from build123d import *

# Parameters (mm, degrees)
BOSS_EXTRUDE1_DEPTH = 60.96
CUT_EXTRUDE1_REACH  = 147.095
SKETCH3_W           = 40.961637843
SKETCH3_H           = 33.750081885


with BuildPart() as part:
    # Sketch1 → Boss-Extrude1 (new body)
    with BuildSketch(Plane(origin=(0, 0, 0), x_dir=(1, 0, 0), z_dir=(0, 1, 0))):
        with BuildLine():
            ThreePointArc((92.976117224, 4.860881604), (-74.724124634, 55.538200742), (22.152321734, -90.429315965))
            ThreePointArc((22.152321734, -90.429315965), (24.083056487, -17.899569011), (92.976117224, 4.860881604))
        make_face()
    extrude(amount=BOSS_EXTRUDE1_DEPTH)

    # Sketch3 → Cut-Extrude1 (cut, up to next)
    with BuildSketch(Plane(origin=(0, 60.96, 0), x_dir=(1, 0, 0), z_dir=(0, 1, 0)), mode=Mode.PRIVATE) as cut_extrude1_sk1:
        with Locations((-100.15988625, -50.336660589)):
            Rectangle(SKETCH3_W, SKETCH3_H)
    cut_extrude1_tool1 = extrude(cut_extrude1_sk1.sketch, amount=-CUT_EXTRUDE1_REACH, mode=Mode.PRIVATE) & part.part
    add(cut_extrude1_tool1.solids().sort_by_distance((-100.159886, 60.96, 50.336661))[0], mode=Mode.SUBTRACT)


solid = part.part
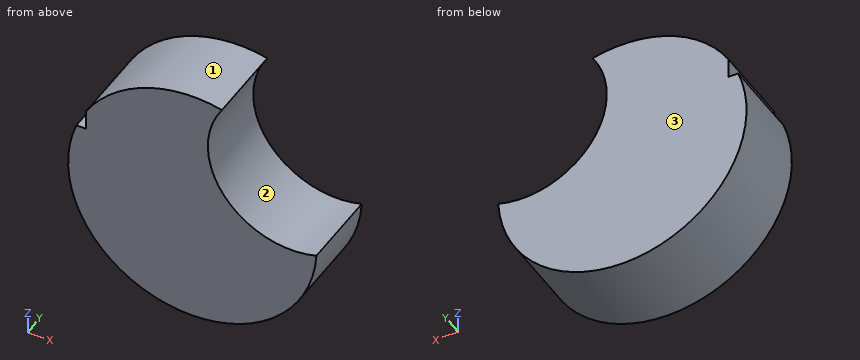
Work out the finished part from the listing and answer in its coordinate system (mm). Face numbers are marked on the shaded views. Give positions to 0.01 mm unless a question says otherwise; leave off trailing zeros. Order: outer loops, then holes, each group sorted by start corner. A loop starts at its lowest first (then second) coordinate and runs counter-clockwise, first axis right, second up. Notation, with made-up numbers: (74.25, -34) -> (86.25, -34) arc R20 ccw to (86.25, -15) -> close; hole circle Ø5 at (82.5, 67). An arc over 180 degrees is marked (long way). Answer as a JSON object with one key per item and string values. Group by question number.
1. The mould has two halves that part along Z. Classify the marked faces 1, 2 and 3: released by +Z, released by -Z, zero draft, split by the parting line, or undercut.
2. Section B-B on x = -62 is taken. Determine the outline of the cut face in (y, z).
3. Section A-A on z = -64 is taken. Determine the outline of the cut face in (x, y).
4. Flat-ended cylindrical pins translate along their axes: pin 1 Ø5 at (y, z) = (12, -58.5) entering from -X; pin 2 Ø8 at (x, y) = (-84, 40.5) entering from +Z; pin 3 Ø1 at (y, z) = (41.5, 16.5) entering from -X. Find the tip coordinate at first contact, or state that the pin passes through.
5. Section C-C on y = 50 is taken. Determine the outline of the cut face in (x, z), plus the area to 3 significant figures.
6. Consider line 1 along Z through (x, y) = (-1, 44.5); line 2 along X through (y, z) = (23.5, 55.5); line 3 along X through (y, z) = (10, -78). Determine where each line is inside the solid, lowest interval first. Write a range as [from, to].
Result sheet:
{
 "1": {"face 1": "released by +Z", "face 2": "undercut", "face 3": "zero draft"},
 "2": {"outline": "(0, -69.46) -> (60.96, -69.46) -> (60.96, 69.46) -> (0, 69.46) -> close"},
 "3": {"outline": "(-67.62, 0) -> (67.62, 0) -> (67.62, 60.96) -> (-67.62, 60.96) -> close"},
 "4": {"pin 1": "stops at x = -74.38", "pin 2": "stops at z = 33.46", "pin 3": "stops at x = -91.72"},
 "5": {"outline": "(-86.88, 33.46) arc R93.1 ccw (long way) to (92.98, -4.86) arc R63.1 cw to (22.15, 90.43) arc R93.1 ccw to (-79.68, 48.16) -> (-79.68, 33.46) -> close", "area": "21,800 mm^2"},
 "6": {"line 1": "z = [-93.1, 93.1]", "line 2": "x = [-74.75, 11.63]", "line 3": "x = [-50.83, 50.83]"}
}
